Read the model definition and answer for the solid it produces. Units are mm, in the model's axes. A direction names the side the tool comes from. Give positions to 0.01 mm unless a question says otherwise; leave off trailing zeros. Loops run counter-clockwise (first coordinate to the right, second up) from the corner with the lowest first, then second, coordinate; pieces in that order, holes last.
(1) Each of these flat-tipped pins is pushed along its axis until it touches: P1, Ø4, axis at x = 0, z = 0, coming from the +Y side; P2, Ø8, axis at x = 6, y = 19.5, coming from the +Z side; P3, Ø5, axis at y = 9.5, z = 8, coming from the +X side. Where does it stop, or does it pass through?
(2) Find section A-A, the plane z = 0. Write down the section's boundary in (x, y).
(3) Find section D-D, the plane z = 30. Write down the section's boundary in (x, y), then the cut area to 3 significant figures.
(4) Find section B-B, the plane y = 4.5. Write down the section's boundary in (x, z).
(5) Find section C-C, the plane x = 30. Write down the section's boundary in (y, z).
(6) Straight lines are drawn through the part: probe 1 along X at (y, z) = (27.9, 0); probe 2 along Z at (x, y) = (-2, 6.5); probe 3 along X at (y, z) = (19, 0). For each, find the intervals that lie inside material, in ascending order.
(7) Which of the six approach directions +Z, -Z, +X, -X, +Y, -Y give full straight-line access (tool end or side, diameter ignored) to faces 1 (the face through (7.37, 14.79, 41.858)), 2 (the face through (0, 25, 0))?
(8) Determine the mould class of faces 3 (the face through (0.1, 14.8, 32.5)), 4 (the face through (-32.565, 14.79, 27.311)), 5 (the face through (-1, 30, 10)) for opening direction Z: pulls with the +Z half, pulls with the -Z half, needs draft (parallel to the pull), parting line crosses it, or undercut.
```python
from build123d import *

# Parameters (mm, degrees)
SALIENTE_EXTRUIR1_DEPTH = 30
CROQUIS2_R              = 2.5
CORTAR_EXTRUIR1_DEPTH   = 5
CROQUIS3_R              = 2.5
CORTAR_EXTRUIR2_DEPTH   = 74.264929004


with BuildPart() as part:
    # Croquis1 → Saliente-Extruir1 (new body)
    with BuildSketch(Plane(origin=(0, 0, 0), x_dir=(1, 0, 0), z_dir=(0, 1, 0))):
        Polygon((-31.838337555, 37.345061187), (-48.260940471, -8.900278543), (-16.422602917, -46.24533973), (31.838337555, -37.345061187), (48.260940471, 8.900278543), (16.422602917, 46.24533973), align=None)
    extrude(amount=SALIENTE_EXTRUIR1_DEPTH)

    # Croquis2 → Cortar-Extruir1 (cut)
    with BuildSketch(Plane(origin=(0, 30, 0), x_dir=(1, 0, 0), z_dir=(0, 1, 0))):
        with Locations(Location((0, 0, 0), (0, 0, 270))):
            Circle(CROQUIS2_R)
    extrude(amount=-CORTAR_EXTRUIR1_DEPTH, mode=Mode.SUBTRACT)

    # Croquis3 → Cortar-Extruir2 (cut, through all)
    with BuildSketch(Plane.XZ):
        with Locations(Location((0, 30, 0), (0, 0, 270))):
            Circle(CROQUIS3_R)
        with Locations(Location((30, 0, 0), (0, 0, 270))):
            Circle(CROQUIS3_R)
    extrude(amount=-CORTAR_EXTRUIR2_DEPTH, mode=Mode.SUBTRACT)


solid = part.part
```
Entries:
1. P1: stops at y = 25
1. P2: stops at z = 42.85
1. P3: stops at x = 43.15
2. outline: (-45.1, 0) - (27.5, 0) - (27.5, 30) - (2.5, 30) - (2.5, 25) - (-2.5, 25) - (-2.5, 30) - (-45.1, 30) - close; (32.5, 0) - (45.1, 0) - (45.1, 30) - (32.5, 30) - close
3. outline: (-30.27, 0) - (-2.5, 0) - (-2.5, 30) - (-30.27, 30) - close; (2.5, 0) - (34.45, 0) - (34.45, 30) - (2.5, 30) - close
3. area: 1,790 mm2
4. outline: (-48.26, 8.9) - (-31.84, -37.35) - (16.42, -46.25) - (48.26, -8.9) - (31.84, 37.35) - (-16.42, 46.25) - close; hole circle Ø5 at (0, 30); hole circle Ø5 at (30, 0)
5. outline: (0, -30.32) - (30, -30.32) - (30, -2.5) - (0, -2.5) - close; (0, 2.5) - (30, 2.5) - (30, 37.68) - (0, 37.68) - close
6. probe 1: x = -45.1 to -2.5, 2.5 to 27.5, 32.5 to 45.1
6. probe 2: z = -42.85 to 28.5, 31.5 to 43.59
6. probe 3: x = -45.1 to 27.5, 32.5 to 45.1
7. face 1: +Z, +X, +Y, -Y
7. face 2: +Y
8. face 3: undercut
8. face 4: pulls with the +Z half
8. face 5: needs draft
